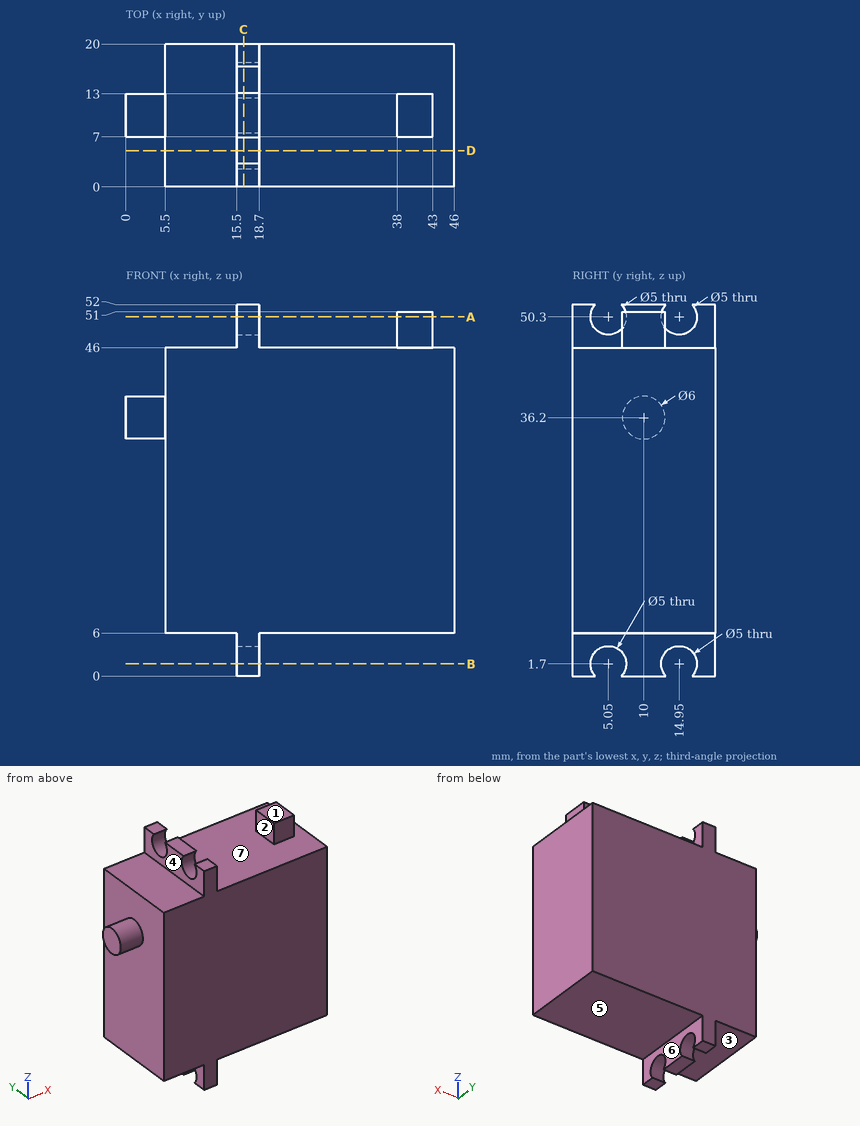
Could you check a few things on this drawing? It's one solid part, dimensions in mm from its lowest x, y, z. A direction names the side the tool comes from. Give positions to 0.01 mm unless a question says otherwise; leave off trailing zeros. Loops run counter-clockwise (first coordinate to the right, second up) from the corner with the lowest first, then second, coordinate; pieces in that order, holes last. Notation, with made-up numbers: (7, 65.5) -> (59, 65.5) arc R8 cw to (59, 78.5) -> close; hole circle Ø3 at (14, -1). An arc over 180 degrees is marked (long way). Use one line per item in the form item = value. Start each with the question number.
1) Which directions (+Z, -Z, +X, -X, +Y, -Y) give clear straight access to the entire face, cutting with the end or side of a thin tool? Please do the marked faces 1, 2, 3 and 4.
2) Please list where these lines run through material, in increasing order: line 1 along Y through (x, z) = (16.95, 50.3); line 2 along Y through (x, z) = (17, 1); line 3 along Z through (x, y) = (17.3, 14.95).
3) For P1, Ø6, axis at x = 28.5, y = 13.5, coming from the -Z side; P2, Ø2.5, axis at x = 39.5, z = 47.5, coming from the +Y side; P3, Ø4, axis at y = 14.95, z = 50.3, coming from the -X side, each with a flat end and sliding along its axis, tell me the tip position at first contact or that it passes through.
4) Imagine slicing it at D-D (y = 5.05). Please give me the cut outline in (x, z).
5) Thinking about a two-plate mould opening in X: for the marked faces 5, 6 and 7, which applies, +X half, -X half, draft (parallel to the pull), parting line (faces both ways), or undercut?
6) Imagine slicing it at B-B (z = 1.7). Please give me the cut outline in (x, y), then the cut area to 3 significant figures.
7) Imagine slicing it at A-A (z = 50.3). Please give me the cut outline in (x, y).
8) Imagine slicing it at C-C (x = 16.5). Please give me the cut outline in (y, z), then the cut area to 3 significant figures.
Check values:
q1.face_1 = +Z, +X, +Y, -Y
q1.face_2 = +Z, +Y, -Y
q1.face_3 = -Z, -X, +Y, -Y
q1.face_4 = +Z, -X, +Y, -Y
q2.line_1 = 0 to 2.55, 7.55 to 12.45, 17.45 to 20
q2.line_2 = 0 to 2.65, 7.45 to 12.55, 17.35 to 20
q2.line_3 = 4.2 to 47.8
q3.P1 = 6
q3.P2 = 13
q3.P3 = 38
q4.outline = (5.5, 6) -> (15.5, 6) -> (15.5, 4.2) -> (18.7, 4.2) -> (18.7, 6) -> (46, 6) -> (46, 46) -> (18.7, 46) -> (18.7, 47.8) -> (15.5, 47.8) -> (15.5, 46) -> (5.5, 46) -> close
q5.face_5 = draft
q5.face_6 = +X half
q5.face_7 = undercut
q6.outline = (15.5, 0) -> (18.7, 0) -> (18.7, 2.55) -> (15.5, 2.55) -> close; (15.5, 7.55) -> (18.7, 7.55) -> (18.7, 12.45) -> (15.5, 12.45) -> close; (15.5, 17.45) -> (18.7, 17.45) -> (18.7, 20) -> (15.5, 20) -> close
q6.area = 32.0 mm^2
q7.outline = (15.5, 0) -> (18.7, 0) -> (18.7, 2.55) -> (15.5, 2.55) -> close; (15.5, 7.55) -> (18.7, 7.55) -> (18.7, 12.45) -> (15.5, 12.45) -> close; (15.5, 17.45) -> (18.7, 17.45) -> (18.7, 20) -> (15.5, 20) -> close; (38, 7) -> (43, 7) -> (43, 13) -> (38, 13) -> close
q8.outline = (0, 0) -> (3.22, 0) arc R2.5 cw (long way) to (6.88, 0) -> (13.12, 0) arc R2.5 cw (long way) to (16.78, 0) -> (20, 0) -> (20, 52) -> (16.78, 52) arc R2.5 cw (long way) to (13.12, 52) -> (6.88, 52) arc R2.5 cw (long way) to (3.22, 52) -> (0, 52) -> close
q8.area = 970 mm^2
